Here's how the part is built. I have some questions about the finished solid (model axes, mm). Face numbers are marked on the shaded views. A direction names the side the tool comes from. Give positions to 0.01 mm unless a question says otherwise; leave off trailing zeros. Write each loop counter-clockwise with the first axis right and the second up, starting at its lowest first coordinate (ties: lowest second). Pieces come first, ordered by that corner, then holes. Notation, with made-up numbers: (83.5, 63.5) -> (127.5, 63.5) arc R14 cw to (127.5, 86.5) -> close; hole circle Ø10 at (81, -25.75). An arc over 180 degrees is marked (long way). Return JSON: item names as keys, results as strings.
from build123d import *

# Parameters (mm, degrees)
F1_DEPTH = 10


with BuildPart() as f1:
    # F0 (on Top) → F1 (new body)
    with BuildSketch(Plane.XY):
        with BuildLine():
            ThreePointArc((-38.901878, 16.278005), (-37.061914, 17.308061), (-36.325796, 19.284071))
            Line((-36.325796, 19.284071), (-37.825796, 19.284071))
            ThreePointArc((-37.825796, 19.284071), (-39.384453, 17.739665), (-40.943111, 19.284071))
            ThreePointArc((-40.943111, 19.284071), (-40.818937, 20.109457), (-40.286706, 20.752427))
            ThreePointArc((-40.286706, 20.752427), (-40.632409, 22.235194), (-41.765545, 21.218282))
            ThreePointArc((-41.765545, 21.218282), (-42.03071, 17.764466), (-38.901878, 16.278005))
        make_face()
        with BuildLine():
            ThreePointArc((-36.325796, 19.284071), (-34.767138, 20.828477), (-33.208481, 19.284071))
            ThreePointArc((-33.208481, 19.284071), (-33.332654, 18.458685), (-33.864885, 17.815715))
            ThreePointArc((-33.864885, 17.815715), (-33.519182, 16.332948), (-32.386046, 17.34986))
            ThreePointArc((-32.386046, 17.34986), (-32.120882, 20.803676), (-35.249713, 22.290136))
            ThreePointArc((-35.249713, 22.290136), (-37.089678, 21.26008), (-37.825796, 19.284071))
            Line((-37.825796, 19.284071), (-36.325796, 19.284071))
        make_face()
    extrude(amount=F1_DEPTH)


solid = f1.part
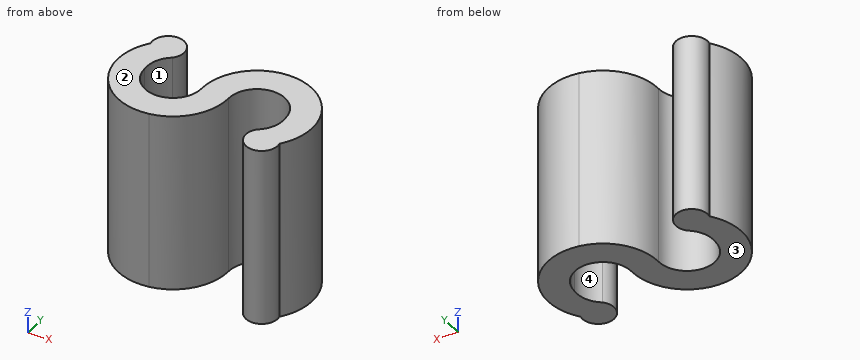
1. For pin 1 Ø2 at (x, z) = (-37.5, 2) entering from -Y; pin 2 Ø1 at (y, z) = (18, 7) entering from +X, each with a flat end and sliding along its axis, tell me the tip position at first contact or that it passes through.
Taken from the geometry:
{"pin 1": "stops at y = 16.37", "pin 2": "stops at x = -31.81"}
2. Suppose I cut it at A-A, the plane x = -33.5. List the corners of the cut face in (y, z) for me.
Taken from the geometry:
{"outline": "(16.33, 0) -> (18.17, 0) -> (18.17, 10) -> (16.33, 10) -> close; (20.18, 0) -> (22.05, 0) -> (22.05, 10) -> (20.18, 10) -> close"}
3. If I drill on line 1 (X direction, y = 18.75, z = 5.25); line 2 (X direction, y = 19.25, z = 6.5); line 3 (X direction, y = 22, z = 4.5), over which ranges is the centre line in solid material (lowest first)? Write a range as [from, to].
Taken from the geometry:
{"line 1": "x = [-42.39, -40.84], [-37.93, -36.38], [-33.24, -31.75]", "line 2": "x = [-42.44, -40.94], [-37.83, -36.33], [-33.2, -31.71]", "line 3": "x = [-41.54, -40.26], [-36.15, -33.39]"}
4. If we mould it in two halves opening along X, with no side actions, what happens to the marked faces 3 and 4? For each: released by +X, released by -X, zero draft, split by the parting line, or undercut.
Taken from the geometry:
{"face 3": "zero draft", "face 4": "undercut"}
5. Which directions (+Z, -Z, +X, -X, +Y, -Y) give clear straight access to the entire face, cutting with the end or side of a thin tool? Please do the marked faces 1 and 2.
Taken from the geometry:
{"face 1": "+Z, -Z", "face 2": "+Z, +X, -X, +Y, -Y"}
6. Suppose I cut it at B-B, the plane y = 19. List the corners of the cut face in (x, z) for me.
Taken from the geometry:
{"outline": "(-42.43, 0) -> (-40.91, 0) -> (-40.91, 10) -> (-42.43, 10) -> close; (-37.85, 0) -> (-36.34, 0) -> (-36.34, 10) -> (-37.85, 10) -> close; (-33.2, 0) -> (-31.72, 0) -> (-31.72, 10) -> (-33.2, 10) -> close"}
7. Suppose I cut it at C-C, the plane y = 21.5. List the corners of the cut face in (x, z) for me, and give its area (3 significant figures).
Taken from the geometry:
{"outline": "(-41.78, 0) -> (-40.02, 0) -> (-40.02, 10) -> (-41.78, 10) -> close; (-36.86, 0) -> (-32.67, 0) -> (-32.67, 10) -> (-36.86, 10) -> close", "area": "59.4 mm²"}
8. Suppose I cut it at D-D, the plane y = 20. List the corners of the cut face in (x, z) for me, and give its area (3 significant figures).
Taken from the geometry:
{"outline": "(-42.36, 0) -> (-40.86, 0) -> (-40.86, 10) -> (-42.36, 10) -> close; (-37.74, 0) -> (-36.14, 0) -> (-36.14, 10) -> (-37.74, 10) -> close; (-33.39, 0) -> (-31.8, 0) -> (-31.8, 10) -> (-33.39, 10) -> close", "area": "46.8 mm²"}
